```python
from build123d import *

# Parameters (mm, degrees)
F0_R     = 40
F0_R_2   = 38
F1_DEPTH = 30
F0_R_3   = 35
F0_R_4   = 30
F2_DEPTH = 5
F3_DEPTH = 3
F4_R     = 39.94757
F4_R_2   = 38
F4_R_3   = 6.844731
F5_DEPTH = 2


with BuildPart() as f1:
    # F0 (on Top) → F1 (new body)
    with BuildSketch(Plane.XY):
        with Locations((-34.639411, 27.720276)):
            Circle(F0_R)
        with Locations((-34.639411, 27.720276)):
            Circle(F0_R_2, mode=Mode.SUBTRACT)
    extrude(amount=F1_DEPTH)

    # F0 (on Top) → F2 (join)
    with BuildSketch(Plane.XY):
        with Locations((-34.639411, 27.720276)):
            Circle(F0_R_2)
        with Locations((-34.639411, 27.720276)):
            Circle(F0_R_3, mode=Mode.SUBTRACT)
        with Locations((-34.639411, 27.720276)):
            Circle(F0_R_3)
        with Locations((-34.639411, 27.720276)):
            Circle(F0_R_4, mode=Mode.SUBTRACT)
    extrude(amount=F2_DEPTH)

    # F0 (on Top) → F3 (cut)
    with BuildSketch(Plane.XY):
        with Locations((-34.639411, 27.720276)):
            Circle(F0_R_3)
        with Locations((-34.639411, 27.720276)):
            Circle(F0_R_4, mode=Mode.SUBTRACT)
    extrude(amount=F3_DEPTH, mode=Mode.SUBTRACT)

    # F4 (on face) → F5 (join)
    with BuildSketch(Plane.XY.offset(30)):
        with Locations((-34.639411, 27.720276)):
            Circle(F4_R)
        with Locations((-34.639411, 27.720276)):
            Circle(F4_R_2, mode=Mode.SUBTRACT)
        with Locations((-34.639411, 27.720276)):
            Circle(F4_R_2)
        with Locations((-34.639411, 27.720276)):
            Circle(F4_R_3, mode=Mode.SUBTRACT)
    extrude(amount=-F5_DEPTH)


solid = f1.part
```
The listing builds one solid part. Answer for the finished solid, in the listing's coordinates (mm). A direction names the side the tool comes from. Coordinates: 2 decimals unless noted, no trailing zeros. Loops run counter-clockwise (first coordinate to the right, second up) from the corner with the lowest first, then second, coordinate; pieces in that order, holes last. Notation, with made-up numbers: M 53.25,72.25 L 62.25,72.25 A16 cw 62.25,87.25 Z; hole C 48.5,84 d9. An arc over 180 degrees is marked long. Answer as a JSON object with one key per item and string values. Group by question number.
Item 1: Section A-A (x = -34) is taken. Write down the section's boundary in (y, z).
Item 2: Section C-C (y = 23.5) is taken. Write down the section's boundary in (x, z).
Item 3: Determine the mould class of faces 1 (the face through (-6.7, 39.2, 5)), 2 (the face through (-8.88, 43.44, 3)), 3 (the face through (-35, 20, 28)), 4 (the face through (3.51, 39.74, 14.79)) for opening direction Z: +Z half, -Z half, draft (parallel to the pull), parting line (faces both ways), or undercut.
Item 4: Section D-D (x = -18) is taken. Write down the section's boundary in (y, z), and give its area (3 significant figures).
Item 5: Each of these flat-tipped pins is pushed along its axis until it touches: P1, Ø5, axis at y = 58.5, z = 7, coming from the -X side; P2, Ø6, axis at x = -54, z = 12.5, coming from the +Y side; P3, Ø1, axis at y = -4, z = 15.5, coming from the -X side. Where does it stop, or does it pass through?
Item 6: Which of the six approach directions +Z, -Z, +X, -X, +Y, -Y give full straight-line access (tool end or side, diameter ignored) to faces 5 (the face through (-41.143, -1.566, 3.986)), 6 (the face through (-35, 19, 30)), 7 (the face through (-64.795, 4.598, 16.339))?
Item 7: Section B-B (y = 59) is taken. Write down the section's boundary in (x, z), and give its area (3 significant figures).
Item 8: Consider L1, parallel to Z at x = -15, y = 20; L2, parallel to X at y = 16, z = 14.5 (3 decimals); L3, parallel to Z at x = -45.5, y = 57.5. Determine where each line is inside the solid, lowest interval first.
Solved:
{
 "1": {"outline": "M -12.27,0 L -7.27,0 L -7.27,3 L -2.27,3 L -2.27,5 L -10.27,5 L -10.27,28 L 20.91,28 L 20.91,30 L -12.27,30 Z; M 34.54,28 L 65.71,28 L 65.71,5 L 57.71,5 L 57.71,3 L 62.71,3 L 62.71,0 L 67.72,0 L 67.72,30 L 34.54,30 Z"},
 "2": {"outline": "M -74.42,0 L -69.38,0 L -69.38,3 L -64.34,3 L -64.34,5 L -72.4,5 L -72.4,28 L -40.03,28 L -40.03,30 L -74.42,30 Z; M -29.25,28 L 3.13,28 L 3.13,5 L -4.94,5 L -4.94,3 L 0.11,3 L 0.11,0 L 5.14,0 L 5.14,30 L -29.25,30 Z"},
 "3": {"face 1": "undercut", "face 2": "-Z half", "face 3": "undercut", "face 4": "draft"},
 "4": {"outline": "M -8.65,0 L -3.07,0 L -3.07,3 L 2.76,3 L 2.76,5 L -6.44,5 L -6.44,28 L 61.88,28 L 61.88,5 L 52.68,5 L 52.68,3 L 58.51,3 L 58.51,0 L 64.1,0 L 64.1,30 L -8.65,30 Z", "area": "326 mm2"},
 "5": {"P1": "stops at x = -62.93", "P2": "stops at y = 64.22", "P3": "stops at x = -59.65"},
 "6": {"face 5": "-Z", "face 6": "+Z, +X, -X, +Y, -Y", "face 7": "none"},
 "7": {"outline": "M -59.57,0 L -50.34,0 L -50.34,3 L -18.94,3 L -18.94,0 L -9.71,0 L -9.71,30 L -59.57,30 Z; hole M -56.22,5 L -13.06,5 L -13.06,28 L -56.22,28 Z", "area": "409 mm2"},
 "8": {"L1": "z = 28 to 30", "L2": "x = -72.884 to -70.787, 1.508 to 3.605", "L3": "z = 3 to 5, 28 to 30"}
}
